The listing builds one solid part. Answer for the finished solid, in the listing's coordinates (mm). A direction names the side the tool comes from. Coordinates: 2 decimals unless noted, no trailing zeros. Order: outer loops, then holes, each group sorted by start corner. A loop starts at its lowest first (then second) coordinate and runs counter-clockwise, first axis right, second up. Notation, with made-up numbers: (35, 36) -> (48, 36) arc R30 cw to (48, 60) -> close; hole circle Ø2 at (77, -40). An arc over 180 degrees is marked (long way). Write each question's results on one line, items separated by ' | '. Start each with the question number.
(1) Determine the mould class of faces 1 (the face through (10.094, -0.046, -33.429)), 2 (the face through (-3.12, -1.8, 14.8)), 3 (the face through (-1.8, 0.38, -45.88)), 4 (the face through (-6.17, -0.05, -36.1)) for opening direction X: +X half, -X half, draft (parallel to the pull), parting line (faces both ways), or undercut.
(2) Given pin 1 (1.1 mm diameter, centred on y = -1, z = -20.5, fed in from +X); pin 2 (2.5 mm diameter, centred on y = -1, z = -20.5, fed in from -X); pin 3 (1.4 mm diameter, centred on y = -1.5, z = -37.5, fed in from +X), each flat-ended and moving along its own axis, determine where each tip first touches the part or whether it passes through.
(3) A tool of negligible diameter and unlimited length cuts with its end or side. For faces 5 (the face through (-3.12, 1.8, 14.8)), 6 (the face through (2.02, -1.8, 14.93)), 7 (the face through (-3.69, -1.76, -20.11)), from which of +Z, -Z, +X, -X, +Y, -Y can it reach the whole face along a straight path? Write none if from no direction.
(4) The part is cut by section A-A, the plane z = -10. Give the vertices of the cut face in (x, y).
(5) Straight lines are drawn through the part: L1, parallel to Z at x = -7.75, y = -0.25; L2, parallel to Y at x = 10.25, z = -30.5; L3, parallel to Z at x = -4.25, y = -2.5. For each, find the intervals that lie inside material, in ascending order.
```python
from build123d import *

# Parameters (mm, degrees)
F2_DEPTH     = 3.2512
F3_DEPTH     = 3.048
F4_T1_DEPTH  = 29.734621701
F4_T3_DEPTH  = 78.5599474126
F4_T5_DEPTH  = 29.3779460523
F4_T7_DEPTH  = 78.2899783824
F4_T10_ANGLE = 237.1999890444
F4_T12_ANGLE = 237.1999890444
F4_T14_ANGLE = 359.64
F4_T16_ANGLE = 359.64


# Not quite as in the source:
# - a fillet or chamfer that OpenCascade refuses, or shapes differently, is made with other operations: its cross-section is extruded or revolved along the edge and cut away or added


with BuildPart() as f1:
    # F0 (on Front) → F1 (revolve)
    with BuildSketch(Plane.XZ):
        with BuildLine():
            Line((-0.6275566491, -35.2181914225), (-3.9520729807, -35.2304723177))
            Line((-3.9520729807, -35.2304723177), (-4.0009869263, -35.190757364))
            ThreePointArc((-4.0009869263, -35.190757364), (-4.468403987, -36.7762535495), (-4.0009869263, -38.361749735))
            ThreePointArc((-4.0009869263, -38.361749735), (-2.9483659374, -38.9416202329), (-1.7635652912, -39.1428866466))
            Line((-1.7635652912, -39.1428866466), (-1.9475727458, -52.4323270698))
            Line((-1.9475727458, -52.4323270698), (-0.5639669494, -52.4323270698))
            Line((-0.5639669494, -52.4323270698), (-0.6275566491, -35.2181914225))
        make_face()
        with BuildLine():
            Line((-0.540195615, -58.8673782805), (-0.5639669494, -52.4323270698))
            Line((-0.5639669494, -52.4323270698), (-1.9475727458, -52.4323270698))
            ThreePointArc((-1.9475727458, -52.4323270698), (-2.3123844436, -52.9312298771), (-2.5166937266, -53.5145388027))
            ThreePointArc((-2.5166937266, -53.5145388027), (-3.6060607732, -55.2257600565), (-2.6693845284, -57.0251033684))
            ThreePointArc((-2.6693845284, -57.0251033684), (-2.3283302078, -57.2524646389), (-1.9475727458, -57.4042373379))
            Line((-1.9475727458, -57.4042373379), (-1.4987547765, -58.7614909788))
            Line((-1.4987547765, -58.7614909788), (-0.820128771, -59.2534937938))
            ThreePointArc((-0.820128771, -59.2534937938), (-0.6865028844, -59.3212967141), (-0.5384338847, -59.3442898632))
            Line((-0.5384338847, -59.3442898632), (-0.540195615, -58.8673782805))
        make_face()
    revolve(axis=Axis((-0.5851411479, 0, -46.7003370305), (0.0036940145, 0, -0.9999931771)))

    # F0 (on Front) → F2 (join, symmetric)
    with BuildSketch(Plane.XZ):
        with BuildLine():
            Line((2.2831694857, -30.7255659779), (-3.495863406, -30.9279132634))
            ThreePointArc((-3.495863406, -30.9279132634), (-5.0646851839, -31.7977900116), (-6.3840295188, -33.0131985247))
            Line((-6.3840295188, -33.0131985247), (-7.2957654484, -31.3216894865))
            Line((-7.2957654484, -31.3216894865), (-8.075539954, -30.6498836726))
            Line((-8.075539954, -30.6498836726), (-8.9392894879, -30.8778174222))
            Line((-8.9392894879, -30.8778174222), (-9.8150353879, -30.2420016378))
            Line((-9.8150353879, -30.2420016378), (-11.11066062, -30.3739625961))
            Line((-11.11066062, -30.3739625961), (-12.0343929157, -29.6901613474))
            Line((-12.0343929157, -29.6901613474), (-13.4499836713, -29.7861322761))
            ThreePointArc((-13.4499836713, -29.7861322761), (-13.6378178947, -29.8303732109), (-13.7259028852, -30.0020705909))
            ThreePointArc((-13.7259028852, -30.0020705909), (-11.3193803546, -33.6661550155), (-8.0515462905, -36.5881621838))
            Line((-8.0515462905, -36.5881621838), (-8.0515462905, -38.0517393351))
            ThreePointArc((-8.0515462905, -38.0517393351), (-7.9598069948, -38.2180289535), (-7.775626611, -38.1717048585))
            Line((-7.775626611, -38.1717048585), (-7.4828979958, -38.2224339632))
            ThreePointArc((-7.4828979958, -38.2224339632), (-6.1405359903, -36.0725037485), (-3.9553394628, -34.7883496227))
            Line((-3.9553394628, -34.7883496227), (-3.9520729807, -35.2304723177))
            Line((-3.9520729807, -35.2304723177), (-0.6275566491, -35.2181914225))
            Line((-0.6275566491, -35.2181914225), (2.6969596825, -35.2059105274))
            Line((2.6969596825, -35.2059105274), (2.6969596825, -34.7637757659))
            ThreePointArc((2.6969596825, -34.7637757659), (4.8915838758, -36.0317506602), (6.2497928845, -38.1717048585))
            ThreePointArc((6.2497928845, -38.1717048585), (6.5108954494, -38.4328074234), (6.7719980143, -38.1717048585))
            Line((6.7719980143, -38.1717048585), (6.7719980143, -36.4611186087))
            ThreePointArc((6.7719980143, -36.4611186087), (10.1347132538, -33.3799368553), (12.5336479489, -29.500936068))
            Line((12.5336479489, -29.500936068), (10.7419602573, -29.0980264544))
            Line((10.7419602573, -29.0980264544), (9.8929585313, -30.0165999209))
            Line((9.8929585313, -30.0165999209), (8.7400143966, -29.6748578548))
            Line((8.7400143966, -29.6748578548), (7.6542128809, -30.5570717901))
            Line((7.6542128809, -30.5570717901), (6.6702044569, -30.3195528686))
            Line((6.6702044569, -30.3195528686), (6.1612352729, -30.8963861316))
            Line((6.1612352729, -30.8963861316), (5.1093655638, -32.7286757529))
            ThreePointArc((5.1093655638, -32.7286757529), (3.7630618873, -31.6328804159), (2.2831694857, -30.7255659779))
        make_face()
    extrude(amount=F2_DEPTH, both=True)

    # F0 (on Front) → F3 (join, symmetric)
    with BuildSketch(Plane.XZ):
        with BuildLine():
            Line((-4.411068745, 48.9967949688), (-4.411068745, -18.4586253017))
            ThreePointArc((-4.411068745, -18.4586253017), (-4.5385726522, -19.078284844), (-4.9003679305, -19.5972640067))
            Line((-4.9003679305, -19.5972640067), (-4.9003679305, -21.9385232776))
            ThreePointArc((-4.9003679305, -21.9385232776), (-3.7434702801, -22.6334289507), (-3.4073905554, -23.9404700696))
            Line((-3.4073905554, -23.9404700696), (-3.4073905554, -26.6549736261))
            Line((-3.4073905554, -26.6549736261), (-3.495863406, -30.9279132634))
            Line((-3.495863406, -30.9279132634), (2.2831694857, -30.7255659779))
            Line((2.2831694857, -30.7255659779), (2.2591357119, -26.7228353769))
            Line((2.2591357119, -26.7228353769), (2.2591357119, -23.9404700696))
            ThreePointArc((2.2591357119, -23.9404700696), (2.5697152514, -22.5087595302), (3.7181819789, -21.5992107987))
            Line((3.7181819789, -21.5992107987), (3.7181819789, -19.3597450852))
            ThreePointArc((3.7181819789, -19.3597450852), (3.4148052065, -18.8087864436), (3.3097744472, -18.1886562715))
            Line((3.3097744472, -18.1886562715), (3.3097744472, 48.9967949688))
            Line((3.3097744472, 48.9967949688), (0, 60.2619871497))
            Line((0, 60.2619871497), (-4.411068745, 48.9967949688))
        make_face()
    extrude(amount=F3_DEPTH, both=True)

    # F4: chamfer of 2.54 on 8 edges, made by hand

    # F4_s2 → F4_t1 (cut)
    with BuildSketch(Plane(origin=(22.8412726569, 0, 58.3331027043), x_dir=(0, 1, 0), z_dir=(-0.3646108065, 0, -0.9311600076))):
        Polygon((3.048, -19.4321717346), (0.508, -21.9721717346), (3.048, -21.9721717346), align=None)
        Polygon((-3.048, -19.4321717346), (-0.508, -21.9721717346), (-3.048, -21.9721717346), align=None)
    extrude(amount=F4_T1_DEPTH, mode=Mode.SUBTRACT)

    # F4_s4 → F4_t3 (cut)
    with BuildSketch(Plane.XY.offset(-18.4586253017)):
        Polygon((-1.871068745, -3.048), (-4.411068745, -0.508), (-4.411068745, -3.048), align=None)
        Polygon((-1.871068745, 3.048), (-4.411068745, 0.508), (-4.411068745, 3.048), align=None)
    extrude(amount=F4_T3_DEPTH, mode=Mode.SUBTRACT)

    # F4_s6 → F4_t5 (cut)
    with BuildSketch(Plane(origin=(-9.8583580644, 0, 33.5540381846), x_dir=(0, 1, 0), z_dir=(-0.2818905922, 0, 0.9594465561))):
        Polygon((3.048, -14.4472872435), (0.508, -16.9872872435), (3.048, -16.9872872435), align=None)
        Polygon((-3.048, -14.4472872435), (-0.508, -16.9872872435), (-3.048, -16.9872872435), align=None)
    extrude(amount=F4_T5_DEPTH, mode=Mode.SUBTRACT)

    # F4_s8 → F4_t7 (cut)
    with BuildSketch(Plane.XY.offset(-18.1886562715)):
        Polygon((0.7697744472, 3.048), (3.3097744472, 0.508), (3.3097744472, 3.048), align=None)
        Polygon((0.7697744472, -3.048), (3.3097744472, -0.508), (3.3097744472, -3.048), align=None)
    extrude(amount=F4_T7_DEPTH, mode=Mode.SUBTRACT)

    # F4_s9 → F4_t10 (revolve, cut)
    with BuildSketch(Plane(origin=(11.9511811184, 0, -7.702013887), x_dir=(0, 1, 0), z_dir=(-0.8405664999, 0, 0.541708371))):
        Polygon((-3.048, 8.0524604286), (-0.508, 10.5924604286), (-3.048, 10.5924604286), align=None)
    revolve(axis=Axis((5.1929984357, -3.048, -18.1886562715), (0, 1, 0)), revolution_arc=F4_T10_ANGLE, mode=Mode.SUBTRACT)

    # F4_s11 → F4_t12 (revolve, cut)
    with BuildSketch(Plane(origin=(11.9511811184, 0, -7.702013887), x_dir=(0, 1, 0), z_dir=(-0.8405664999, 0, 0.541708371))):
        Polygon((3.048, 8.0524604286), (0.508, 10.5924604286), (3.048, 10.5924604286), align=None)
    revolve(axis=Axis((5.1929984357, 3.048, -18.1886562715), (0, 1, 0)), revolution_arc=F4_T12_ANGLE, mode=Mode.SUBTRACT)

    # F4_s13 → F4_t14 (revolve, cut)
    with BuildSketch(Plane.XY.offset(-18.4586253017)):
        Polygon((-1.871068745, 3.048), (-4.411068745, 0.508), (-4.411068745, 3.048), align=None)
    revolve(axis=Axis((-5.9805704311, 3.048, -18.4586253017), (0, 1, 0)), revolution_arc=F4_T14_ANGLE, mode=Mode.SUBTRACT)

    # F4_s15 → F4_t16 (revolve, cut)
    with BuildSketch(Plane.XY.offset(-18.4586253017)):
        Polygon((-1.871068745, -3.048), (-4.411068745, -0.508), (-4.411068745, -3.048), align=None)
    revolve(axis=Axis((-5.9805704311, -3.048, -18.4586253017), (0, 1, 0)), revolution_arc=F4_T16_ANGLE, mode=Mode.SUBTRACT)


solid = f1.part
```
Established:
1) face 1: +X half | face 2: -X half | face 3: parting line | face 4: undercut
2) pin 1: stops at x = 3.72 | pin 2: stops at x = -4.9 | pin 3: stops at x = 6.77
3) face 5: +Z, -X, +Y | face 6: +Z, +X, -Y | face 7: +Z, -X, -Y
4) outline: (-4.41, -0.51) -> (-1.87, -3.05) -> (0.77, -3.05) -> (3.31, -0.51) -> (3.31, 0.51) -> (0.77, 3.05) -> (-1.87, 3.05) -> (-4.41, 0.51) -> close
5) L1: z = -38.18 to -30.93 | L2: y = -3.25 to 3.25 | L3: z = -34.89 to -31.29, -22.17 to -21.57
